Geometry: final body of the model. Coordinates: model frame, mm. A direction names the side the tool comes from. Round coordinates to 2 decimals unless told otherwise and drop trailing zeros. Loops run counter-clockwise (first coordinate to the right, second up) from the corner with the lowest first, then second, coordinate; pieces in that order, holes last. Notation, with made-up numbers: (79, -19.5) - (104, -19.5) arc R13 cw to (104, -1.5) - close; hole circle Ø6 at (-30.5, 25). An arc over 180 degrees is marked (long way). Answer in a Markdown table with one row per item. Add a question column.
Autodesk Inventor part; units mm, degrees
ref_plane "YZ Plane" through (0, 0, 0) normal (1, 0, 0) x (0, 1, 0)
ref_plane "XZ Plane" through (0, 0, 0) normal (0, 1, 0) x (-1, 0, 0)
ref_plane "XY Plane" through (0, 0, 0) normal (0, 0, 1) x (1, 0, 0)
sketch "Sketch1" plane through (0, 0, 0) normal (0, 0, 1) x (1, 0, 0)
  circle A0 centre (0, 0) radius 18.0975
  dimension "d0" = 36.195
extrude "Extrusion1" add sketch "Sketch1" along normal blind 17.78
sketch "Sketch2" plane through (0, 0, 17.78) normal (0, 0, 1) x (1, 0, 0)
  circle A0 centre (0, 0) radius 18.0975
  line L0 (0, -18.0975) -> (0, -6.6929) construction
  circle A1 centre (0, -6.6929) radius 5.969
  dimension "d3" = 11.4046
  dimension "d4" = 11.938
extrude "Extrusion2" add sketch "Sketch2" along normal blind 4.318 contours A1
sketch "Sketch3" plane through (0, -6.6929, 22.098) normal (0, 0, 1) x (1, 0, 0)
  circle A0 centre (0, 0) radius 5.969
  circle A1 centre (0, 0) radius 3
  point P0 (0, 6.6929)
  dimension "d7" = 6
extrude "Extrusion3" add sketch "Sketch3" along normal blind 18.415 contours A1
sketch "Sketch4" plane through (0, -6.6929, 40.513) normal (0, 0, 1) x (1, 0, 0)
  circle A0 centre (0, 0) radius 3
  arc A1 (1.6583, 2.5) -> (-1.6583, 2.5) centre (0, 0) ccw
  line L0 (-1.6583, 2.5) -> (1.6583, 2.5)
  point P0 (0, 6.6929)
extrude "Extrusion4" cut sketch "Sketch4" against normal blind 12 contours L0 A0 picked at (-0.1169, 2.6598)
sketch "Sketch5" plane through (0, 0, 0) normal (0, 0, -1) x (-1, 0, 0)
  circle A0 centre (0, 0) radius 18.0975
  circle A1 centre (0, 0) radius 16.51
  dimension "d13" = 33.02
extrude "Extrusion5" add sketch "Sketch5" along normal blind 22.86 contours A1
sketch "Sketch6" plane through (0, 0, -22.86) normal (0, 0, -1) x (-1, 0, 0)
  circle A0 centre (0, 0) radius 16.51
  circle A1 centre (0, 0) radius 4.445
  dimension "d16" = 8.89
extrude "Extrusion6" add sketch "Sketch6" along normal blind 3.175 contours A1
sketch "Sketch7" plane through (0, 0, 17.78) normal (0, 0, 1) x (1, 0, 0)
  circle A0 centre (0, 0) radius 18.0975
  circle A1 centre (-15.494, 0) radius 1.5
  circle A2 centre (15.494, 0) radius 1.5
  circle A3 centre (0, 0) radius 15.494 construction
  circle A4 centre (15.494, 0) radius 26.8478 construction
  circle A5 centre (-7.7668, 13.4068) radius 26.8478 construction
  circle A6 centre (-7.7668, 13.4068) radius 1.5
  circle A7 centre (-7.747, -13.441) radius 1.5
  dimension "d24" = 53.6956
  dimension "d21" = 3
  dimension "d22" = 3
  dimension "d23" = 53.6956
  dimension "d25" = 3
  dimension "d26" = 3
extrude "Extrusion7" cut sketch "Sketch7" against normal blind 12.7 contours A1 | A2 | A6 | A7
thread "Thread1"
thread "Thread2"
thread "Thread3"
thread "Thread4"
properties part number "Drive Motor"
1) Section A-A, the plane x = 0. Return the cut outline in (y, z) (1 decimal).
2) Section B-B, the plane y = 0. Return the cut outline in (x, z) (1 decimal).
3) Section D-D, the plane x = -12.5. Return the cut outline in (y, z), and give its area (3 significant figures).
4) Pull-direction query (Y, two-part tool) for faces 4 (the flat face through (-3.4, -3.4, -22.86)), 5 (the cylindrical face through (-1.294, -0.866, 19.909)), 6 (the cylindrical face through (13.995, 0.066, 11.519)), 7 (the cylindrical face through (-7.05, -14.77, 11.52)); classes: pulls with the +Y half, pulls with the -Y half, needs draft (parallel to the pull), parting line crosses it, or undercut.
5) Reachability of faces 1 (the flat face through (15, -8, 0)), 2 (the flat face through (0, -4.193, 35)), 3 (the flat face through (-8, -13, 5.08)) from +Z, -Z, +X, -X, +Y, -Y: full face, straight path, thin tool, end or side. Return the list, or none.
6) Material intervals for line 1 along X through (y, z) = (0.5, 11); line 2 along Z through (x, y) = (4.5, 6); line 3 along Y through (x, z) = (15.5, 6.5), sorted ascending. Write a range as from..to.
7) Section C-C, the plane z = -7. Return the cut outline in (x, y).
8) Contact query for flat-ended pins moving along their axis: pin 1 Ø3.5 at (x, z) = (-0.5, 32) entering from +Y; pin 2 Ø1.5 at (x, y) = (-3, -10.5) entering from -Z; pin 3 Ø0.9 at (x, y) = (-7.5, -13) entering from +Z; pin 4 Ø12 at (y, z) = (1.5, 7.5) entering from -X. Output: stop coordinate, or through.
Evaluation:
| question | item | result |
|---|---|---|
| 1 | outline | (-18.1, 0) - (-16.5, 0) - (-16.5, -22.9) - (-4.4, -22.9) - (-4.4, -26) - (4.4, -26) - (4.4, -22.9) - (16.5, -22.9) - (16.5, 0) - (18.1, 0) - (18.1, 17.8) - (-0.7, 17.8) - (-0.7, 22.1) - (-3.7, 22.1) - (-3.7, 28.5) - (-4.2, 28.5) - (-4.2, 40.5) - (-9.7, 40.5) - (-9.7, 22.1) - (-12.7, 22.1) - (-12.7, 17.8) - (-18.1, 17.8) - close |
| 2 | outline | (-18.1, 0) - (-16.5, 0) - (-16.5, -22.9) - (-4.4, -22.9) - (-4.4, -26) - (4.4, -26) - (4.4, -22.9) - (16.5, -22.9) - (16.5, 0) - (18.1, 0) - (18.1, 17.8) - (17, 17.8) - (17, 5.1) - (14, 5.1) - (14, 17.8) - (-14, 17.8) - (-14, 5.1) - (-17, 5.1) - (-17, 17.8) - (-18.1, 17.8) - close |
| 3 | outline | (-13.09, 0) - (-10.79, 0) - (-10.79, -22.86) - (10.79, -22.86) - (10.79, 0) - (13.09, 0) - (13.09, 17.78) - (-13.09, 17.78) - close |
| 3 | area | 958 mm² |
| 4 | face 4 | needs draft |
| 4 | face 5 | parting line crosses it |
| 4 | face 6 | undercut |
| 4 | face 7 | undercut |
| 5 | face 1 | -Z |
| 5 | face 2 | +Z, +X, -X, +Y |
| 5 | face 3 | +Z |
| 6 | line 1 | x = -18.09..-16.91, -14.08..14.08, 16.91..18.09 |
| 6 | line 2 | z = -22.86..17.78 |
| 6 | line 3 | y = -9.34..-1.5, 1.5..9.34 |
| 7 | outline | circle Ø33.02 at (0, 0) |
| 8 | pin 1 | stops at y = -4.19 |
| 8 | pin 2 | stops at z = -22.86 |
| 8 | pin 3 | stops at z = 5.08 |
| 8 | pin 4 | stops at x = -18.1 |
